Input: part model. Units: mm. Frame: model coordinates. Face numbers are marked on the shaded views. A direction names the side the tool comes from. Give positions to 0.01 mm unless a question says otherwise; leave off trailing zeros. Write each loop counter-clockwise with the first axis right and the second up, starting at its lowest first coordinate (ties: lowest second). Pieces come first, ordered by that corner, then holes. Notation, with made-up numbers: (46.5, 76.25) - (68.5, 76.25) arc R18 ccw to (68.5, 92.25) - close; hole circle Ø4 at (22, 20). An arc over 180 degrees is marked (long way). Answer as CSV lines item,"result".
```python
from build123d import *

# Parameters (mm, degrees)
SKETCH1_W           = 20
SKETCH1_H           = 30
BOSS_EXTRUDE1_DEPTH = 10
FILLET1_R           = 4


with BuildPart() as part:
    # Sketch1 → Boss-Extrude1 (new body)
    with BuildSketch(Plane(origin=(0, 0, 0), x_dir=(1, 0, 0), z_dir=(0, 1, 0))):
        Rectangle(SKETCH1_W, SKETCH1_H)
        with BuildLine():
            Line((1.7, 10.8), (1.7, 3.2))
            ThreePointArc((1.7, 3.2), (0, 1.5), (-1.7, 3.2))
            Line((-1.7, 3.2), (-1.7, 10.8))
            ThreePointArc((-1.7, 10.8), (0, 12.5), (1.7, 10.8))
        make_face(mode=Mode.SUBTRACT)
        with BuildLine():
            Line((1.7, -10.8), (1.7, -3.2))
            ThreePointArc((1.7, -3.2), (0, -1.5), (-1.7, -3.2))
            Line((-1.7, -3.2), (-1.7, -10.8))
            ThreePointArc((-1.7, -10.8), (0, -12.5), (1.7, -10.8))
        make_face(mode=Mode.SUBTRACT)
    extrude(amount=BOSS_EXTRUDE1_DEPTH)

    # Fillet1
    fillet1_edges = [part.edges().sort_by_distance(p)[0] for p in [
        (10, 5, 15),
        (-10, 5, 15),
        (-10, 5, -15),
        (10, 5, -15),
    ]]
    fillet(fillet1_edges, radius=FILLET1_R)


solid = part.part
```
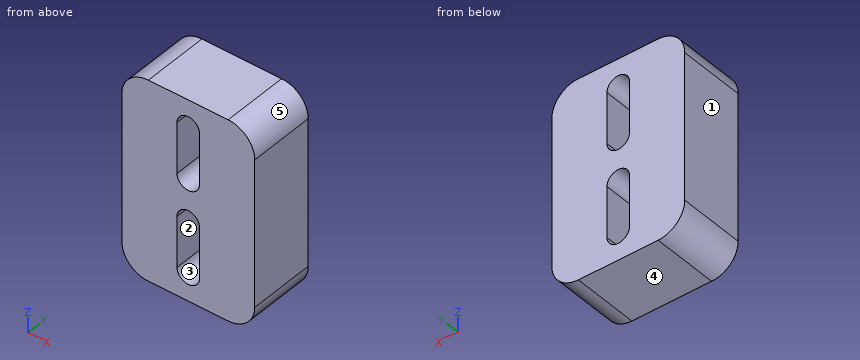
Item 1: Ray query, line 1 (X direction, y = 6.75, z = -5.5); line 2 (Z direction, x = 0.75, y = 4); line 3 (Z direction, x = 1.25, y = 6). Return the intervals inside material, ascending. Write a range as from..to.
The answers:
line 1,"-10..-1.7, 1.7..10"
line 2,"-15..-12.33, -1.67..1.67, 12.33..15"
line 3,"-15..-11.95, -2.05..2.05, 11.95..15"
Item 2: Cut plane B-B on z = 7.5. Return the cut outline in (x, y), plus the area to 3 significant figures.
The answers:
outline,"(-10, 0) - (-1.7, 0) - (-1.7, 10) - (-10, 10) - close; (1.7, 0) - (10, 0) - (10, 10) - (1.7, 10) - close"
area,"166 mm²"
Item 3: Mould query, pull axis X, two halves, no side actions, for the marked faces 3, 4 and 5. Classes: +X half, -X half, draft (parallel to the pull), parting line (faces both ways), or undercut.
The answers:
face 3,"undercut"
face 4,"draft"
face 5,"+X half"
Item 4: Contact query for a flat-ended pin moving along its axis: pin 1 (1 mm diameter, centred on x = 0, z = -5.5, fed in from +Y). Output: stop coordinate, or through.
The answers:
pin 1,"through"
Item 5: Cut plane C-C on x = 0. Return the cut outline in (y, z), plus the area to 3 significant figures.
The answers:
outline,"(0, -15) - (10, -15) - (10, -12.5) - (0, -12.5) - close; (0, -1.5) - (10, -1.5) - (10, 1.5) - (0, 1.5) - close; (0, 12.5) - (10, 12.5) - (10, 15) - (0, 15) - close"
area,"80.0 mm²"
Item 6: Cut plane A-A on y = 8.25. Return the cut outline in (x, z).
The answers:
outline,"(-10, -11) arc R4 ccw to (-6, -15) - (6, -15) arc R4 ccw to (10, -11) - (10, 11) arc R4 ccw to (6, 15) - (-6, 15) arc R4 ccw to (-10, 11) - close; hole (-1.7, -10.8) arc R1.7 ccw to (1.7, -10.8) - (1.7, -3.2) arc R1.7 ccw to (-1.7, -3.2) - close; hole (-1.7, 3.2) arc R1.7 ccw to (1.7, 3.2) - (1.7, 10.8) arc R1.7 ccw to (-1.7, 10.8) - close"
Item 7: Reachability of the marked faces 1 and 2 from +Z, -Z, +X, -X, +Y, -Y: full face, straight path, thin tool, end or side. Return the list, or none.
The answers:
face 1,"+Z, -Z, -X, +Y, -Y"
face 2,"+Y, -Y"
